from build123d import *

# Parameters (mm, degrees)
PAD007_DEPTH           = 20
SKETCH020_W            = 1
SKETCH020_H            = 9
POCKET012_DEPTH        = 275
SKETCH033_R            = 1.5
POCKET021_DEPTH        = 120.5
LINEARPATTERN005_COUNT = 14
LINEARPATTERN005_PITCH = 21.153846


with BuildPart() as part:
    # Sketch019 → Pad007 (new body)
    with BuildSketch(Plane.XY):
        Polygon((0, 275), (0, 0), (-20, 0), (-20, 275), (-255, 275), (-255, 0), (-275, 0), (-275, 295), (0, 295), align=None)
    extrude(amount=PAD007_DEPTH)

    # Sketch020 → Pocket012 (cut)
    with BuildSketch(Plane.XZ):
        with Locations((-19.5, 10)):
            Rectangle(SKETCH020_W, SKETCH020_H)
        with Locations((-255.5, 10)):
            Rectangle(SKETCH020_W, SKETCH020_H)
    extrude(amount=-POCKET012_DEPTH, mode=Mode.SUBTRACT)

    # Sketch033 → Pocket021 (cut, symmetric)
    with BuildSketch(Plane(origin=(-137.5, 1, 0), x_dir=(0, 1, 0), z_dir=(1, 0, 0))):
        with Locations((266.5, 10)):
            Circle(SKETCH033_R)
    pocket021 = extrude(amount=POCKET021_DEPTH, both=True, mode=Mode.SUBTRACT)

    # LinearPattern005: Pocket021 ×14
    with Locations(*[(0, -i * LINEARPATTERN005_PITCH, 0) for i in range(1, LINEARPATTERN005_COUNT)]):
        add(pocket021, mode=Mode.SUBTRACT)


solid = part.part
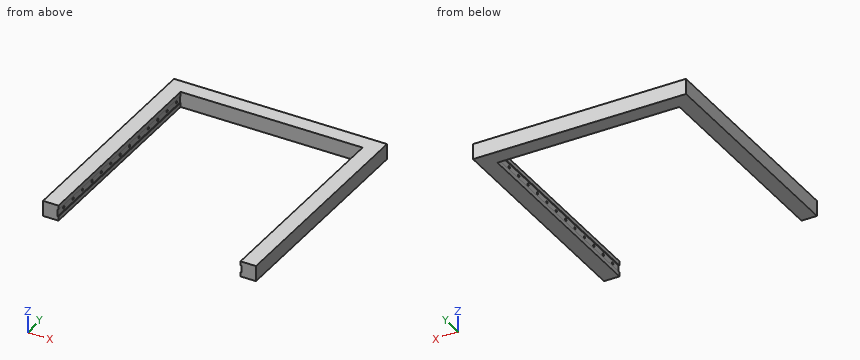
Verification items for the finished model (mm, model axes). Coordinates: 2 decimals unless noted, no trailing zeros. Order: outer loops, then holes, each group sorted by start corner. A loop starts at its lowest first (then second) coordinate and runs counter-clockwise, first axis right, second up.
Item 1: Section check B-B, the plane x = -130.5. Enter the section's corners in (y, z), then the cut area to 3 significant figures.
Filled in:
outline: (275, 0) - (295, 0) - (295, 20) - (275, 20) - close
area: 400 mm2
Item 2: Section check A-A, the plane y = 105.5. Enter the section's corners in (x, z), then the cut area to 3 significant figures.
Filled in:
outline: (-275, 0) - (-255, 0) - (-255, 5.5) - (-256, 5.5) - (-256, 14.5) - (-255, 14.5) - (-255, 20) - (-275, 20) - close; (-20, 0) - (0, 0) - (0, 20) - (-20, 20) - (-20, 14.5) - (-19, 14.5) - (-19, 5.5) - (-20, 5.5) - close
area: 782 mm2
Item 3: Material ranges on L1, parallel to X at y = 176, z = 6.75; L2, parallel to X at y = 222, z = 1.5; L3, parallel to Y at x = -192.5, z = 12.5, recorded low to high.
Filled in:
L1: x = -275 to -256, -19 to 0
L2: x = -275 to -255, -20 to 0
L3: y = 275 to 295
Item 4: Depth check by flat-ended pin: pin 1 (8 mm diameter, centred on x = -136.5, z = 13.5, fed in from -Y). Enter the tip coordinate at first touch or a pass-through.
Filled in:
pin 1: stops at y = 275
